Verification items for the finished model (mm, model axes). A direction names the side the tool comes from. Round coordinates to 2 decimals unless told otherwise and drop trailing zeros. Loops run counter-clockwise (first coordinate to the right, second up) from the corner with the lowest first, then second, coordinate; pieces in that order, holes last. Notation, with made-up numbers: (34.25, 51.25) -> (46.25, 51.25) arc R5 ccw to (46.25, 58.25) -> close; hole circle Ø8 at (-0.5, 38). An arc over 180 degrees is marked (long way). Write item = value, one per line.
```python
from build123d import *

# Parameters (mm, degrees)
CHAMFER_1_SIZE      = 0.3
CHAMFER_1_SIZE2     = 0.519615242
FILLET_1_R          = 0.4
FILLET_2_SIZE       = 0.5
FILLET_2_SIZE_2     = 0.8
CUT_EXTRUDE_1_DEPTH = 2


with BuildPart() as part:
    # 草图2 → 旋转1 (revolve)
    with BuildSketch(Plane(origin=(0, 0, 0), x_dir=(0, 0, -1), z_dir=(1, 0, 0)), mode=Mode.PRIVATE) as revolve_1_sk:
        Polygon((-9.5, 0), (-9.5, 3.4), (-5.5, 3.4), (-5.5, 2), (9.5, 2), (9.5, 0), align=None)
    revolve(revolve_1_sk.sketch.rotate(Axis((0, 0, -9.5), (0, 0, 1)), 90), axis=Axis((0, 0, -9.5), (0, 0, 1)))

    # 倒角1
    chamfer_1_edges = [part.edges().sort_by_distance(p)[0] for p in [
        (2, 0, -9.5),
    ]]
    chamfer_1_side = [part.faces().sort_by_distance(p)[0] for p in [
        (2, 0, -2),
    ]]
    chamfer(chamfer_1_edges, length=CHAMFER_1_SIZE, length2=CHAMFER_1_SIZE2, reference=chamfer_1_side[0])

    # 圆角1
    fillet_1_edges = [part.edges().sort_by_distance(p)[0] for p in [
        (3.4, 0, 5.5),
    ]]
    fillet(fillet_1_edges, radius=FILLET_1_R)

    # 圆角2
    # an asymmetric fillet: 0.8, 0.5 mm, written as the material it takes off along each edge
    with BuildSketch(Plane(origin=(0, 0, 9.5), x_dir=(-1, 0, 0), z_dir=(0, 1, 0))) as fillet_2_piece_1:
        with BuildLine():
            Bezier((3.4, -FILLET_2_SIZE), (3.4, 0), (3.4 - FILLET_2_SIZE_2, 0), weights=[1, 0.707106781, 1])
            Line((3.4 - FILLET_2_SIZE_2, 0), (3.4, 0))
            Line((3.4, 0), (3.4, -FILLET_2_SIZE))
        make_face()
    revolve(axis=Axis((0, 0, 9.5), (0, 0, 1)), mode=Mode.SUBTRACT)

    # 草图3 → 切除-拉伸1 (cut)
    with BuildSketch(Plane.XY.offset(9.5)):
        Polygon((0, 1.732050808), (-1.5, 0.866025404), (-1.5, -0.866025404), (0, -1.732050808), (1.5, -0.866025404), (1.5, 0.866025404), align=None)
    extrude(amount=-CUT_EXTRUDE_1_DEPTH, mode=Mode.SUBTRACT)


solid = part.part
```
(1) Set-up check for faces 5 (the face through (-1, 2, 5.5)), 6 (the face through (0, 0, 7.5)), 7 (the face through (0, 0, -9.5)): record each of +Z, -Z, +X, -X, +Y, -Y from which the full face is reachable in a straight line by a thin tool's end or side.
Filled sheet:
face_5 = -Z
face_6 = +Z
face_7 = -Z, +X, -X, +Y, -Y
(2) Go/stop test with flat-tipped pins: pin 1 Ø4 at (x, y) = (-1.5, -1) entering from -Z; pin 2 Ø3 at (y, z) = (2, -4) entering from +X; pin 3 Ø1.5 at (y, z) = (-1, -0.5) entering from +X; pin 4 Ø4 at (x, z) = (2, 3) entering from +Y. Record where each tip stops, or that it passes through.
Filled sheet:
pin_1 = -9.5
pin_2 = 1.94
pin_3 = 1.98
pin_4 = 2
(3) Material ranges on probe 1 along X at (y, z) = (1, -0.75); probe 2 along Z at (x, y) = (0.75, 0.75), recorded low to high. Write a range as from..to.
Filled sheet:
probe_1 = -1.73..1.73
probe_2 = -9.5..7.5
(4) Sectioned sample at A-A, the plane z = 2.5. Record the cut outline in (x, y), and give its area (3 significant figures).
Filled sheet:
outline = circle Ø4 at (0, 0)
area = 12.6 mm2
(5) Draft check along X on faces 1 (the face through (-1.5, 0, 9)), 2 (the face through (0.74, 3.32, 7.43)), 3 (the face through (2, 0, 9.5)), 4 (the face through (-0.76, -1.293, 8.514)). Enter one of: released by +X, released by -X, zero draft, split by the parting line, or undercut.
Filled sheet:
face_1 = undercut
face_2 = split by the parting line
face_3 = zero draft
face_4 = undercut
